Study the drawing (mm; zero at the part's minimum x, y, z) and answer. A direction names the side the tool comes from. Coordinates: 2 decimals unless noted, no trailing zeros. Order: outer loops, then holes, each group sorted by start corner. A loop starts at its lowest first (then second) coordinate and runs counter-clockwise, first axis right, second up. Notation, with made-up numbers: (22, 47) -> (67, 47) arc R16 ccw to (67, 73) -> close; hole circle Ø10 at (60.25, 81). An arc over 180 degrees is marked (long way). Write each question's results on one line, items separated by ' | '. Start each with the question number.
(1) Straight lines are drawn through the part: L1, parallel to Z at x = 34, y = 2.25; L2, parallel to Y at x = 19, z = 43.2 (1 decimal); L3, parallel to Y at x = 30, z = 40 (1 decimal). For each, find the intervals that lie inside material, in ascending order.
(2) A tool of negligible diameter and unlimited length cuts with its end or side. For the marked faces 1 and 2, from which of +Z, -Z, +X, -X, +Y, -Y can it reach the whole face along a straight path? Write none if from no direction.
(3) The part is cut by section A-A, the plane z = 4. Count the separate pieces of the cut face and the enclosed holes in it, then the cut area to 3 significant figures.
(4) The part is cut by section B-B, the plane x = 19. Give the vertices of the cut face in (y, z) (1 decimal).
(5) Given pin 1 (4 mm diameter, centred on x = 34, z = 34, fed in from -Y); pin 2 (5 mm diameter, centred on x = 23.5, z = 38, fed in from +Y) (3 decimals); pin 3 (10 mm diameter, centred on x = 24.5, y = 33.5, fed in from -Z) (3 decimals), each flat-ended and moving along its own axis, determine where each tip first touches the part or whether it passes through.
(6) The part is cut by section D-D, the plane x = 6.5. Give the vertices of the cut face in (y, z) (1 decimal).
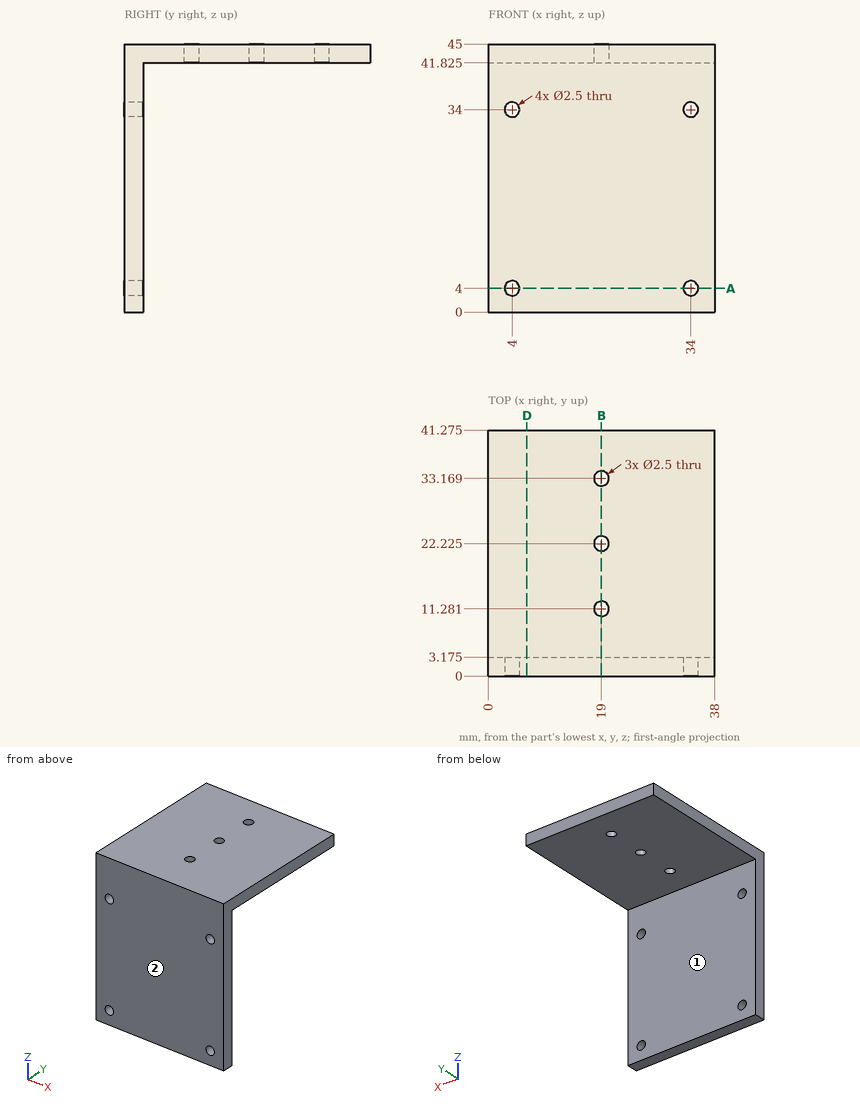
Established:
1) L1: z = 0 to 2.75, 5.25 to 32.75, 35.25 to 45 | L2: y = 0 to 10, 12.5 to 21, 23.5 to 31.9, 34.4 to 41.3 | L3: y = 0 to 3.2
2) face 1: -Z, +X, -X, +Y | face 2: +Z, -Z, +X, -X, -Y
3) separate pieces: 3 | enclosed holes: 0 | area: 105 mm^2
4) outline: (0, 0) -> (3.2, 0) -> (3.2, 41.8) -> (10, 41.8) -> (10, 45) -> (0, 45) -> close; (12.5, 41.8) -> (21, 41.8) -> (21, 45) -> (12.5, 45) -> close; (23.5, 41.8) -> (31.9, 41.8) -> (31.9, 45) -> (23.5, 45) -> close; (34.4, 41.8) -> (41.3, 41.8) -> (41.3, 45) -> (34.4, 45) -> close
5) pin 1: stops at y = 0 | pin 2: stops at y = 3.175 | pin 3: stops at z = 41.825
6) outline: (0, 0) -> (3.2, 0) -> (3.2, 41.8) -> (41.3, 41.8) -> (41.3, 45) -> (0, 45) -> close
